Build history of the part. All positions in model axes, mm. Give positions to 0.01 mm unless a question says otherwise; leave off trailing zeros. Order: outer loops, then holes, each group sorted by start corner. A loop starts at its lowest first (then second) coordinate and runs counter-clockwise, first axis right, second up. Notation, with made-up numbers: (20.25, -36.75) - (47.25, -36.75) arc R12 ccw to (47.25, -20.75) - close; hole circle Ø11 at (-20.5, 60). An arc over 180 degrees is marked (long way). Use a Markdown table: item, result.
from build123d import *

# Parameters (mm, degrees)
EXTRUDE_1_DEPTH     = 4
SKETCH_2_R          = 5
CUT_EXTRUDE_1_DEPTH = 5


with BuildPart() as part:
    # Эскиз1 → Бобышка-Вытянуть1 (new body)
    with BuildSketch(Plane(origin=(0, 0, 0), x_dir=(1, 0, 0), z_dir=(0, 1, 0))):
        with BuildLine():
            Line((0, 0), (10, 0))
            ThreePointArc((10, 0), (17.071067812, 2.928932188), (20, 10))
            Line((20, 10), (20, 20))
            Line((20, 20), (10, 20))
            ThreePointArc((10, 20), (2.928932188, 17.071067812), (0, 10))
            Line((0, 10), (0, 0))
        make_face()
    extrude(amount=EXTRUDE_1_DEPTH)

    # Эскиз2 → Вырез-Вытянуть1 (cut, through all)
    with BuildSketch(Plane(origin=(0, 4, 0), x_dir=(1, 0, 0), z_dir=(0, 1, 0))):
        with Locations((10, 10)):
            Circle(SKETCH_2_R)
    extrude(amount=-CUT_EXTRUDE_1_DEPTH, mode=Mode.SUBTRACT)


solid = part.part
1) Two-plate mould, pull along Z, no slides. Class faces 1 (the cylindrical face through (14.77, 2.03, -11.5)), 2 (the flat face through (5, 2, 0)), 3 (the flat face through (20, 2, -15)): +Z half, -Z half, draft (parallel to the pull), parting line (faces both ways), or undercut.
Computed:
| item | result |
|---|---|
| face 1 | undercut |
| face 2 | +Z half |
| face 3 | draft |
2) Slice it at B-B (z = -5.75). Write the cut outline in (x, y), and give its area (3 significant figures).
Computed:
| item | result |
|---|---|
| outline | (0, 0) - (7.37, 0) - (7.37, 4) - (0, 4) - close; (12.63, 0) - (19.05, 0) - (19.05, 4) - (12.63, 4) - close |
| area | 55.1 mm² |
3) Slice it at D-D (x = 18). Write the cut outline in (y, z).
Computed:
| item | result |
|---|---|
| outline | (0, -20) - (4, -20) - (4, -4) - (0, -4) - close |
4) Slice it at A-A (y = 0.5). Write the cut outline in (x, z).
Computed:
| item | result |
|---|---|
| outline | (0, -10) arc R10 ccw to (10, -20) - (20, -20) - (20, -10) arc R10 ccw to (10, 0) - (0, 0) - close; hole circle Ø10 at (10, -10) |
5) Wall check: line 1 (X direction, y = 2.3, z = -10); line 2 (Z direction, x = 10, y = 1.8); line 3 (Z direction, x = 11.25, y = 0.3). Give the ranges that are in metal, low to high. Write a range as from..to.
Computed:
| item | result |
|---|---|
| line 1 | x = 0..5, 15..20 |
| line 2 | z = -20..-15, -5..0 |
| line 3 | z = -20..-14.84, -5.16..-0.08 |
6) Pin check, flat tip, straight feed: P1, Ø1.5, axis at x = 2.5, y = 2, coming from the -Z side. Stop position of the tip, or through.
Computed:
| item | result |
|---|---|
| P1 | stops at z = -17.38 |
7) Slice it at C-C (x = 12.25). Write the cut outline in (y, z), and give its area (3 significant figures).
Computed:
| item | result |
|---|---|
| outline | (0, -20) - (4, -20) - (4, -14.47) - (0, -14.47) - close; (0, -5.53) - (4, -5.53) - (4, -0.26) - (0, -0.26) - close |
| area | 43.3 mm² |
